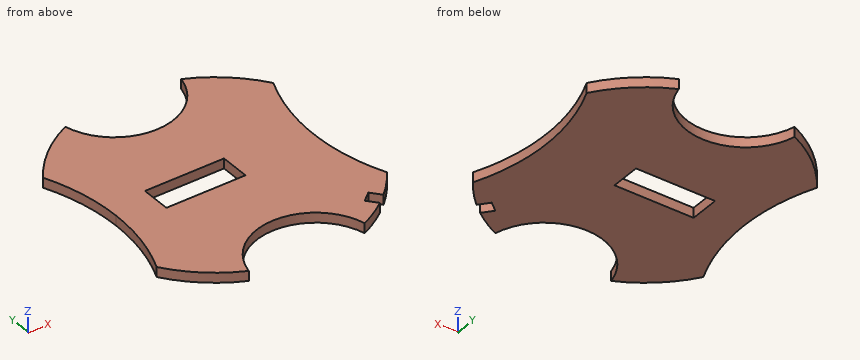
from build123d import *

# Parameters (mm, degrees)
F0_R     = 70.5
F1_DEPTH = 5
F2_W     = 40
F2_H     = 15
F3_DEPTH = 25
F5_DEPTH = 25
F7_DEPTH = 25


with BuildPart() as f1:
    # F0 (on Top) → F1 (new body)
    with BuildSketch(Plane.XY):
        Circle(F0_R)
    extrude(amount=F1_DEPTH)

    # F2 (on face) → F3 (cut)
    with BuildSketch(Plane.XY.offset(5)):
        with Locations((-10, 0)):
            Rectangle(F2_W, F2_H)
    extrude(amount=-F3_DEPTH, mode=Mode.SUBTRACT)

    # F4 (on face) → F5 (cut)
    with BuildSketch(Plane.XY.offset(5)):
        with BuildLine():
            ThreePointArc((29.3130957529, 64.1170212766), (0, 70.5), (-29.3130957529, 64.1170212766))
            ThreePointArc((-29.3130957529, 64.1170212766), (0, 40.5), (29.3130957529, 64.1170212766))
        make_face()
        with BuildLine():
            ThreePointArc((-50, 0), (-52.0801773558, 20.2905971655), (-58.2341666667, 39.7370335158))
            ThreePointArc((-58.2341666667, 39.7370335158), (-70.5, 0), (-58.2341666667, -39.7370335158))
            ThreePointArc((-58.2341666667, -39.7370335158), (-52.0801773558, -20.2905971655), (-50, 0))
        make_face()
        with BuildLine():
            ThreePointArc((29.3130957529, -64.1170212766), (0, -40.5), (-29.3130957529, -64.1170212766))
            ThreePointArc((-29.3130957529, -64.1170212766), (0, -70.5), (29.3130957529, -64.1170212766))
        make_face()
        with BuildLine():
            ThreePointArc((70.5, 0), (67.363783853, 20.7935236312), (58.2341666667, 39.7370335158))
            ThreePointArc((58.2341666667, 39.7370335158), (50, 0), (58.2341666667, -39.7370335158))
            ThreePointArc((58.2341666667, -39.7370335158), (67.363783853, -20.7935236312), (70.5, 0))
        make_face()
    extrude(amount=-F5_DEPTH, mode=Mode.SUBTRACT)

    # F6 (on face) → F7 (cut)
    with BuildSketch(Plane.XY.offset(5)):
        with BuildLine():
            ThreePointArc((42.9773455668, -55.88557746), (45.3165264829, -54.0061332399), (47.5736122255, -52.0288518018))
            Line((47.5736122255, -52.0288518018), (43.4365403493, -47.0984815306))
            Line((43.4365403493, -47.0984815306), (38.8402736906, -50.9552071887))
            Line((38.8402736906, -50.9552071887), (42.9773455668, -55.88557746))
        make_face()
    extrude(amount=-F7_DEPTH, mode=Mode.SUBTRACT)


solid = f1.part
Verification items for the finished model (mm, model axes). Give positions to 0.01 mm unless a question says otherwise; leave off trailing zeros. Order: outer loops, then holes, each group sorted by start corner. A loop starts at its lowest first (then second) coordinate and runs counter-clockwise, first axis right, second up. Notation, with made-up numbers: M 46.25,65 L 61.25,65 A14 cw 61.25,90 Z; hole C -34.75,59.5 d3. An arc over 180 degrees is marked long. Answer as a JSON object with one key per item and string values. Group by question number.
1) Cross-section at C-C (y = 51). Enter the section's corners in (x, z), then the cut area to 3 significant figures.
2) Depth check by flat-ended pin: pin 1 Ø1.5 at (x, z) = (-0.5, 4) entering from -Y; pin 2 Ø1.5 at (y, z) = (21, 2) entering from -X; pin 3 Ø2 at (y, z) = (-7.5, 2.5) entering from -X. Enter the tip coordinate at first touch or a pass-through.
3) Cross-section at B-B (z = 1.3). Enter the section's corners in (x, y).
4) Cross-section at D-D (x = 36.5). Enter the section's corners in (y, z).
5) Cross-section at A-A (x = -20.5). Enter the section's corners in (y, z).
6) Scan lines: line 1 along Y through (x, z) = (2, 3.65); line 2 along X through (y, z) = (-59, 0.8); line 3 along X through (y, z) = (52, 2.1). Record each from-to range of solid material in increasing order. Write a range as [from, to].
Result sheet:
{
 "1": {"outline": "M -48.67,0 L -22.8,0 L -22.8,5 L -48.67,5 Z; M 22.8,0 L 48.67,0 L 48.67,5 L 22.8,5 Z", "area": "259 mm2"},
 "2": {"pin 1": "stops at y = -40.53", "pin 2": "stops at x = -52.39", "pin 3": "stops at x = -50.36"},
 "3": {"outline": "M -58.23,-39.74 A70.5 ccw -29.31,-64.12 A30 cw 29.31,-64.12 A70.5 ccw 42.98,-55.89 L 38.84,-50.96 L 43.44,-47.1 L 47.57,-52.03 A70.5 ccw 58.23,-39.74 A100 cw 58.23,39.74 A70.5 ccw 29.31,64.12 A30 cw -29.31,64.12 A70.5 ccw -58.23,39.74 A100 cw Z; hole M -30,-7.5 L 10,-7.5 L 10,7.5 L -30,7.5 Z"},
 "4": {"outline": "M -60.32,0 L 60.32,0 L 60.32,5 L -60.32,5 Z"},
 "5": {"outline": "M -48.6,0 L -7.5,0 L -7.5,5 L -48.6,5 Z; M 7.5,0 L 48.6,0 L 48.6,5 L 7.5,5 Z"},
 "6": {"line 1": "y = [-40.57, -7.5], [7.5, 40.57]", "line 2": "x = [-38.59, -27.71], [27.71, 38.59]", "line 3": "x = [-47.61, -23.62], [23.62, 47.61]"}
}
